Verification items for the finished model (mm, model axes). Round coordinates to 2 decimals unless told otherwise and drop trailing zeros. Loops run counter-clockwise (first coordinate to the right, second up) from the corner with the lowest first, then second, coordinate; pieces in that order, holes last. Notation, with made-up numbers: (6, 68.25) -> (47, 68.25) arc R7 cw to (47, 73.25) -> close; hole circle Ø7 at (89, 74.25). An arc over 180 degrees is marked (long way). Write item = value, one per line. Start each with the question number.
```python
from build123d import *

# Parameters (mm, degrees)
F1_DEPTH = 2.54
F2_R     = 22.86
F3_R     = 29.21
F4_R     = 44.45
F5_R     = 22.86
F6_R     = 27.94
F8_DEPTH = 2.54


with BuildPart() as f1:
    # F0 (on Front) → F1 (new body)
    with BuildSketch(Plane.XZ):
        Polygon((64.1644249716, 70.274220109), (-66.6455750284, 70.274220109), (-66.6455750284, -88.475779891), (-23.4655750284, -88.475779891), (64.1644249716, -2.115779891), align=None)
    extrude(amount=F1_DEPTH)

    # F2
    f2_edges = [f1.edges().sort_by_distance(p)[0] for p in [
        (-66.645575, -1.27, 70.27422),
    ]]
    fillet(f2_edges, radius=F2_R)

    # F3
    f3_edges = [f1.edges().sort_by_distance(p)[0] for p in [
        (64.164425, -1.27, 70.27422),
    ]]
    fillet(f3_edges, radius=F3_R)

    # F4
    f4_edges = [f1.edges().sort_by_distance(p)[0] for p in [
        (64.164425, -1.27, -2.11578),
    ]]
    fillet(f4_edges, radius=F4_R)

    # F5
    f5_edges = [f1.edges().sort_by_distance(p)[0] for p in [
        (-66.645575, -1.27, -88.47578),
    ]]
    fillet(f5_edges, radius=F5_R)

    # F6
    f6_edges = [f1.edges().sort_by_distance(p)[0] for p in [
        (-23.465575, -1.27, -88.47578),
    ]]
    fillet(f6_edges, radius=F6_R)

    # F7 (on face) → F8 (cut, through all)
    with BuildSketch(Plane.XZ.offset(2.54)):
        with BuildLine():
            ThreePointArc((42.8920452321, -7.0321095397), (50.1746073496, 3.7388999191), (52.7344249716, 16.4863580775))
            Line((52.7344249716, 16.4863580775), (52.7344249716, 41.064220109))
            ThreePointArc((52.7344249716, 41.064220109), (47.5267835411, 53.6365786785), (34.9544249716, 58.844220109))
            Line((34.9544249716, 58.844220109), (-43.7855750284, 58.844220109))
            ThreePointArc((-43.7855750284, 58.844220109), (-51.8678055373, 55.4964506179), (-55.2155750284, 47.414220109))
            Line((-55.2155750284, 47.414220109), (-55.2155750284, -65.615779891))
            ThreePointArc((-55.2155750284, -65.615779891), (-51.8678055373, -73.6980104), (-43.7855750284, -77.045779891))
            Line((-43.7855750284, -77.045779891), (-34.9194176486, -77.045779891))
            ThreePointArc((-34.9194176486, -77.045779891), (-28.6570239441, -75.8119877022), (-23.3306075184, -72.2950136996))
            Line((-23.3306075184, -72.2950136996), (42.8920452321, -7.0321095397))
        make_face()
    extrude(amount=-F8_DEPTH, mode=Mode.SUBTRACT)


solid = f1.part
```
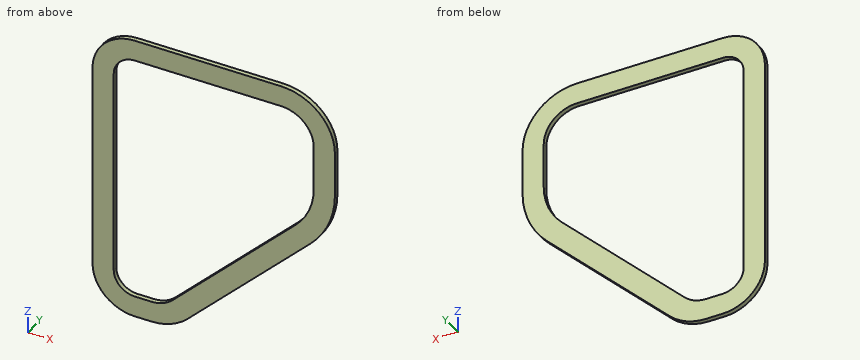
(1) Depth check by flat-ended pin: pin 1 Ø1 at (x, y) = (37, -2.5) entering from -Z; pin 2 Ø1.3 at (x, y) = (10, -1.5) entering from -Z. Enter the tip coordinate at first touch or a pass-through.
(2) Section check A-A on z = 26. Enter the section's corners in (x, y).
(3) Section check D-D on x = -59. Enter the section's corners in (y, z).
(4) Section check B-B on x = -38. Enter the section's corners in (y, z).
(5) Section check C-C on y = -1.3. Enter the section's corners in (x, z), then the cut area to 3 significant figures.
(6) Scan lines: line 1 (X direction, y = -1.7, z = 24.5); line 2 (Z direction, x = -34.5, y = -2.05); line 3 (X direction, y = -2.35, z = -5). Record each from-to range of solid material in increasing order. Write a range as [from, to].
Computed values:
q1.pin_1 = -29.38
q1.pin_2 = -56.14
q2.outline = (-66.65, -2.54) -> (-55.22, -2.54) -> (-55.22, 0) -> (-66.65, 0) -> close; (52.73, -2.54) -> (64.16, -2.54) -> (64.16, 0) -> (52.73, 0) -> close
q3.outline = (-2.54, -82.68) -> (0, -82.68) -> (0, 64.48) -> (-2.54, 64.48) -> close
q4.outline = (-2.54, -88.48) -> (0, -88.48) -> (0, -77.05) -> (-2.54, -77.05) -> close; (-2.54, 58.84) -> (0, 58.84) -> (0, 70.27) -> (-2.54, 70.27) -> close
q5.outline = (-66.65, -65.62) arc R22.86 ccw to (-43.79, -88.48) -> (-34.92, -88.48) arc R27.94 ccw to (-15.31, -80.44) -> (50.92, -15.17) arc R44.45 ccw to (64.16, 16.49) -> (64.16, 41.06) arc R29.21 ccw to (34.95, 70.27) -> (-43.79, 70.27) arc R22.86 ccw to (-66.65, 47.41) -> close; hole (-55.22, -65.62) arc R11.43 ccw to (-43.79, -77.05) -> (-34.92, -77.05) arc R16.51 ccw to (-23.33, -72.3) -> (42.89, -7.03) arc R33.02 ccw to (52.73, 16.49) -> (52.73, 41.06) arc R17.78 ccw to (34.95, 58.84) -> (-43.79, 58.84) arc R11.43 ccw to (-55.22, 47.41) -> close
q5.area = 5,220 mm²
q6.line_1 = [-66.65, -55.22], [52.73, 64.16]
q6.line_2 = [-88.47, -77.04], [58.84, 70.27]
q6.line_3 = [-66.65, -55.22], [44.79, 58.63]
